Input: dimensioned drawing with shaded views. Units: mm. Origin: part minimum x, y, z. A direction names the side the tool comes from. Round coordinates to 2 decimals unless told otherwise and drop trailing zeros. Order: outer loops, then holes, each group sorted by start corner. A loop starts at its lowest first (then second) coordinate and runs counter-clockwise, first axis right, second up. Notation, with made-up numbers: (48.5, -37.5) -> (95.5, -37.5) arc R15 ccw to (95.5, -18.5) -> close; hole circle Ø7 at (80.25, -35.75). An arc over 180 degrees is marked (long way). Use a Markdown table: item, result. Add a question column.
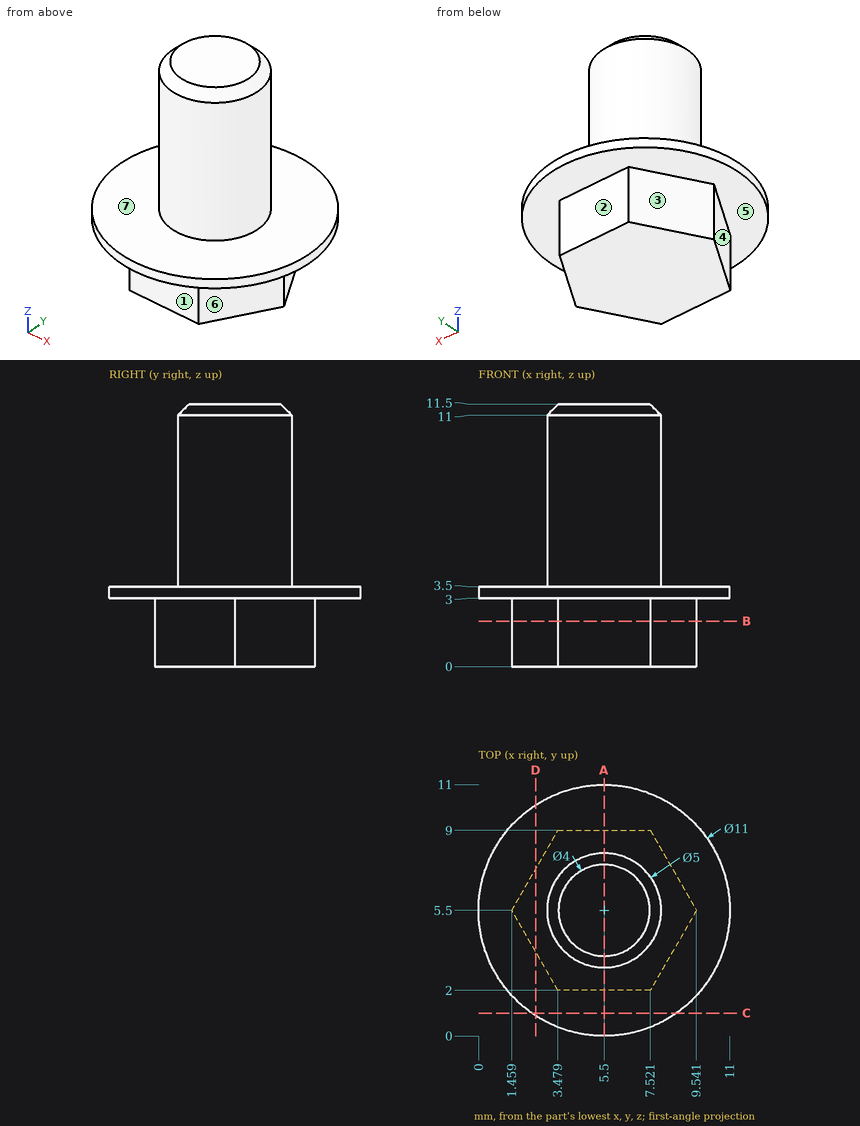
1) Section C-C on y = 1. Output: boundary loops of the cut face in (x, z).
2) First-contact query: pin 1 Ø1.5 at (x, y) = (3, 1.5) entering from +Z; pin 2 Ø1.5 at (y, z) = (7, 9.5) entering from -X (1 decimal); pin 3 Ø0.9 at (x, z) = (6, 1.5) entering from -Y; pin 4 Ø1.5 at (y, z) = (9.5, 7.5) entering from -X. Flat tips, straight axial feed; report the tip coordinate or a pass-through.
3) Draft query along Z for the marked faces 5, 6 and 7. Return one class per face: pulls with the +Z half, pulls with the -Z half, needs draft (parallel to the pull), parting line crosses it, or undercut.
4) Section A-A on x = 5.5. Output: boundary loops of the cut face in (y, z).
5) Line query: probe 1 along Z at (x, y) = (8.75, 6.75); probe 2 along Z at (x, y) = (2.5, 7.5); probe 3 along Y at (x, z) = (4, 7.5). Output: solid intervals per line, ascending. Write a range as from..to.
6) Section B-B on z = 2. Output: boundary loops of the cut face in (x, y).
7) Reachability of the marked faces 1, 2, 3 and 4 from +Z, -Z, +X, -X, +Y, -Y: full face, straight path, thin tool, end or side. Return the list, or none.
8) Section D-D on x = 2.5. Output: boundary loops of the cut face in (y, z).
Conclusion:
| question | item | result |
|---|---|---|
| 1 | outline | (2.34, 3) -> (8.66, 3) -> (8.66, 3.5) -> (2.34, 3.5) -> close |
| 2 | pin 1 | stops at z = 3.5 |
| 2 | pin 2 | stops at x = 3.1 |
| 2 | pin 3 | stops at y = 2 |
| 2 | pin 4 | passes through |
| 3 | face 5 | pulls with the -Z half |
| 3 | face 6 | needs draft |
| 3 | face 7 | pulls with the +Z half |
| 4 | outline | (0, 3) -> (2, 3) -> (2, 0) -> (9, 0) -> (9, 3) -> (11, 3) -> (11, 3.5) -> (8, 3.5) -> (8, 11) -> (7.5, 11.5) -> (3.5, 11.5) -> (3, 11) -> (3, 3.5) -> (0, 3.5) -> close |
| 5 | probe 1 | z = 0..3.5 |
| 5 | probe 2 | z = 3..3.5 |
| 5 | probe 3 | y = 3.5..7.5 |
| 6 | outline | (1.46, 5.5) -> (3.48, 2) -> (7.52, 2) -> (9.54, 5.5) -> (7.52, 9) -> (3.48, 9) -> close |
| 7 | face 1 | -Z, +X, -X, -Y |
| 7 | face 2 | -Z, +X, -X, +Y |
| 7 | face 3 | -Z, -X, +Y |
| 7 | face 4 | -Z, -X, -Y |
| 8 | outline | (0.89, 3) -> (3.7, 3) -> (3.7, 0) -> (7.3, 0) -> (7.3, 3) -> (10.11, 3) -> (10.11, 3.5) -> (0.89, 3.5) -> close |
